Source: CAD feature listing. Evaluate the final solid. Frame: model axes, mm. A direction names the side the tool comes from. Give positions to 0.01 mm unless a question says otherwise; leave off trailing zeros. Write each loop counter-clockwise with the first axis right and the second up, starting at its lowest first coordinate (ties: lowest second). Pieces come first, ordered by that corner, then holes. Notation, with made-up numbers: (47, 32) -> (75, 32) arc R14 ccw to (75, 54) -> close; hole circle Ø5 at (18, -35.75). An arc over 180 degrees is marked (long way). Answer as a JSON object with one key per item and string values. Group by question number.
Item 1: First-contact query: pin 1 Ø5.5 at (x, z) = (-4, 9) entering from -Y; pin 2 Ø1 at (x, z) = (-3.5, 6.5) entering from +Y; pin 3 Ø8 at (x, z) = (-16.5, 19) entering from +Y; pin 4 Ø5 at (x, y) = (17.27, -12.97) entering from -Z. Flat tips, straight axial feed; report the tip coordinate or a pass-through.
Item 2: Section query D-D on x = -19. Give the number of separate pieces and of enclosed holes in the cut face, plus the area to 3 significant figures.
Item 3: Ray query, probe 1 along Z at (x, y) = (-18, -10); probe 2 along X at (y, z) = (-7.5, 2); probe 3 along Y at (x, z) = (27.5, 28.5). Return the intervals inside material, ascending. Write a range as from..to.
Item 4: Pull-direction query (X, two-part tool) for faces 4 (the face through (-2.755, 0.868, 22.288)), 5 (the face through (-16.082, 3.489, 10.92)), 6 (the face through (5, 0, 0)), 7 (the face through (47.495, -1, 9)); classes: pulls with the +X half, pulls with the -X half, needs draft (parallel to the pull), parting line crosses it, or undercut.
Item 5: Section query A-A on x = 0. Return the cut outline in (y, z), plus the area to 3 significant figures.
Item 6: Section query C-C on z = 14. Return the cut outline in (x, y), plus the area to 3 significant figures.
Item 7: Access query for faces 1 (the face through (-37.128, -1, 9)), 2 (the face through (5, -36.658, 9)), 3 (the face through (54.603, 0.108, 27.158)). Directions: +Z, -Z, +X, -X, +Y, -Y. A direction counts if a zero-diameter tool reaches every point of the face in a straight line with its end or side. Return the directions, or none.
Item 8: Section query B-B on z = 28. Return the cut outline in (x, y), plus the area to 3 significant figures.
from build123d import *

# Parameters (mm, degrees)
F0_W           = 84.6236236393
F0_H           = 72.3108425736
F1_DEPTH       = 25
F3_D           = 5.5
F3_CSINK_D     = 11.2
F3_CSINK_ANGLE = 90


with BuildPart() as f1:
    # F0 (on Top) → F1 (new body)
    with BuildSketch(Plane.XY):
        with Locations((5.1834825426, -0.5025528371)):
            Rectangle(F0_W, F0_H)
    extrude(amount=F1_DEPTH)

    # F3 (through all)
    with Locations(Plane.XY.offset(25)):
        with Locations((-18.4712763876, -21.672623232), (17.2712653875, -12.972522527), (0, 0), (-18.829761073, 3.3679855987), (30.8238454163, 16.1767713726)):
            CounterSinkHole(F3_D / 2, F3_CSINK_D / 2, counter_sink_angle=F3_CSINK_ANGLE)

    # F5: sweep along a path in F5_path
    with BuildLine(Plane(origin=(47.4952943623, 35.6528684497, 25), x_dir=(0, -1, 0), z_dir=(0, 0, -1))) as f5_path:
        Line((0, 0), (0, 84.6236236393))
        Line((0, 84.6236236393), (72.3108425736, 84.6236236393))
        Line((72.3108425736, 84.6236236393), (72.3108425736, 0))
        Line((72.3108425736, 0), (0, 0))
    # F4 (on face) → F5 (sweep)
    with BuildSketch(Plane(origin=(-37.128329277, 0, 0), x_dir=(0, -1, 0), z_dir=(-1, 0, 0))):
        with BuildLine():
            Line((-35.6528684497, 25), (-28.2249371945, 25))
            ThreePointArc((-28.2249371945, 25), (-40.9052090104, 30.2523405608), (-35.6528684497, 17.5720687448))
            Line((-35.6528684497, 17.5720687448), (-35.6528684497, 25))
        make_face()
    sweep(path=f5_path.line, transition=Transition.RIGHT)


solid = f1.part
Worked answers:
{
 "1": {"pin 1": "y = -36.66", "pin 2": "y = 35.65", "pin 3": "y = 42.81", "pin 4": "through"},
 "2": {"separate pieces": "3", "enclosed holes": "0", "area": "1,780 mm^2"},
 "3": {"probe 1": "0..25", "probe 2": "-37.13..47.5", "probe 3": "-43.21..-30.11, 29.1..42.2"},
 "4": {"face 4": "undercut", "face 5": "undercut", "face 6": "needs draft", "face 7": "pulls with the +X half"},
 "5": {"outline": "(-36.66, 0) -> (-2.75, 0) -> (-2.75, 22.15) -> (-5.6, 25) -> (-29.23, 25) arc R7.43 ccw (long way) to (-36.66, 17.57) -> close; (2.75, 0) -> (35.65, 0) -> (35.65, 17.57) arc R7.43 ccw (long way) to (28.22, 25) -> (5.6, 25) -> (2.75, 22.15) -> close", "area": "1,920 mm^2"},
 "6": {"outline": "(-37.13, -36.66) -> (47.5, -36.66) -> (47.5, 35.65) -> (-37.13, 35.65) -> close; hole circle Ø5.5 at (-18.83, 3.37); hole circle Ø5.5 at (-18.47, -21.67); hole circle Ø5.5 at (0, 0); hole circle Ø5.5 at (17.27, -12.97); hole circle Ø5.5 at (30.82, 16.18)", "area": "6,000 mm^2"},
 "7": {"face 1": "-Z, -X, +Y, -Y", "face 2": "-Z, +X, -X, -Y", "face 3": "none"},
 "8": {"outline": "(-43.92, -43.45) -> (54.29, -43.45) -> (54.29, 42.45) -> (-43.92, 42.45) -> close; hole (-30.33, -29.86) -> (40.7, -29.86) -> (40.7, 28.86) -> (-30.33, 28.86) -> close", "area": "4,270 mm^2"}
}
